Source: three-view drawing plus pictorial views. Frame: mm from the lowest corner of the part. A direction names the side the tool comes from. Give positions to 0.01 mm unless a question says otherwise; leave off trailing zeros. Loops run counter-clockwise (first coordinate to the right, second up) from the corner with the lowest first, then second, coordinate; pieces in that order, holes last.
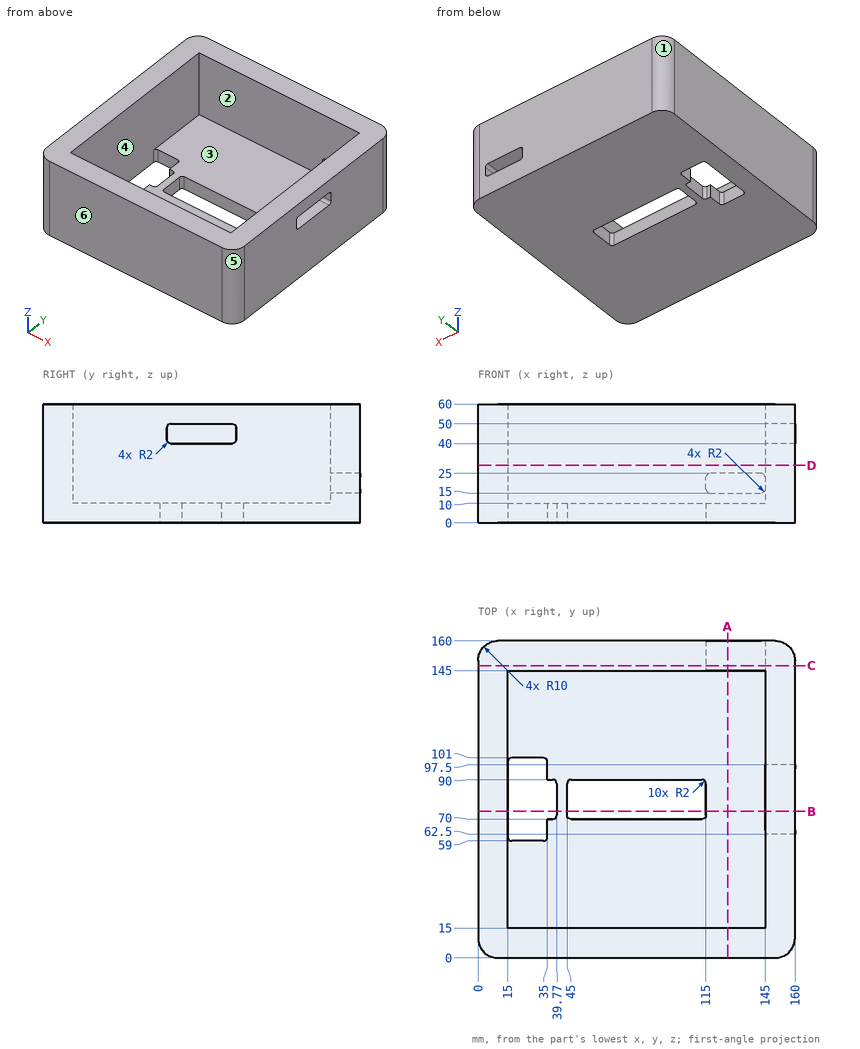
(1) Pin query (flat end, axial travel): pin 1 Ø12 at (x, y) = (22, 24) entering from +Z; pin 2 Ø1.8 at (x, z) = (154, 44.5) entering from -Y. Return the tip coordinate at first contact, or that it passes through.
Values follow:
pin 1: stops at z = 10
pin 2: stops at y = 0.49
(2) Cut plane C-C (y = 147.5). Return the cut outline in (x, z).
Values follow:
outline: (0, 0) - (160, 0) - (160, 60) - (0, 60) - close; hole (115, 17) arc R2 ccw to (117, 15) - (143, 15) arc R2 ccw to (145, 17) - (145, 23) arc R2 ccw to (143, 25) - (117, 25) arc R2 ccw to (115, 23) - close
(3) Cut plane B-B (y = 74). Return the cut outline in (x, z), and give its area (3 significant figures).
Values follow:
outline: (0, 0) - (15, 0) - (15, 60) - (0, 60) - close; (39.77, 0) - (45, 0) - (45, 10) - (39.77, 10) - close; (115, 0) - (160, 0) - (160, 40) - (145, 40) - (145, 10) - (115, 10) - close; (145, 50) - (160, 50) - (160, 60) - (145, 60) - close
area: 2,000 mm2
(4) Reachability of the marked faces 1 and 2 from +Z, -Z, +X, -X, +Y, -Y: full face, straight path, thin tool, end or side. Return the list, or none.
Values follow:
face 1: +Z, -Z, -X, +Y
face 2: +Z
(5) Cut plane A-A (x = 126). Return the cut outline in (y, z), and give its area (3 significant figures).
Values follow:
outline: (0, 0) - (160, 0) - (160, 15) - (145, 15) - (145, 10) - (15, 10) - (15, 60) - (0, 60) - close; (145, 25) - (160, 25) - (160, 60) - (145, 60) - close
area: 2,950 mm2
(6) Ray query, probe 1 along X at (y, z) = (73.5, 54.5); probe 2 along Y at (x, z) = (19, 8). Return the intervals inside material, ascending.
Values follow:
probe 1: x = 0 to 15, 145 to 160
probe 2: y = 0 to 59, 101 to 160
(7) Mould query, pull axis X, two halves, no side actions, for the marked faces 3, 4, 5 and 6. Classes: +X half, -X half, draft (parallel to the pull), parting line (faces both ways), or undercut.
Values follow:
face 3: undercut
face 4: undercut
face 5: +X half
face 6: draft
(8) Cut plane D-D (z = 29). Return the cut outline in (x, y).
Values follow:
outline: (0, 10) arc R10 ccw to (10, 0) - (150, 0) arc R10 ccw to (160, 10) - (160, 150) arc R10 ccw to (150, 160) - (10, 160) arc R10 ccw to (0, 150) - close; hole (15, 15) - (145, 15) - (145, 145) - (15, 145) - close
